```python
from build123d import *

# Parameters (mm, degrees)
BOSS_EXTRU_1_DEPTH = 8


with BuildPart() as part:
    # Esquisse2 → Boss.-Extru.1 (new body)
    with BuildSketch(Plane.XY):
        with BuildLine():
            Line((-234, 77.582220472), (250, 77.582220472))
            Line((250, 77.582220472), (250, 68.582220472))
            Line((250, 68.582220472), (230.972064578, 68.582220472))
            ThreePointArc((230.972064578, 68.582220472), (228.850744234, 68.582220472), (228.850744234, 66.460900128))
            Line((228.850744234, 66.460900128), (228.850744234, 60.582220472))
            Line((228.850744234, 60.582220472), (218.850744234, 60.582220472))
            Line((218.850744234, 60.582220472), (218.850744234, 66.460900128))
            ThreePointArc((218.850744234, 66.460900128), (218.850744234, 68.582220472), (216.729423891, 68.582220472))
            Line((216.729423891, 68.582220472), (115.787517246, 68.582220472))
            ThreePointArc((115.787517246, 68.582220472), (113.666196902, 68.582220472), (113.666196902, 66.460900128))
            Line((113.666196902, 66.460900128), (113.666196902, 60.582220472))
            Line((113.666196902, 60.582220472), (63.666196902, 60.582220472))
            Line((63.666196902, 60.582220472), (63.666196902, 66.460900128))
            ThreePointArc((63.666196902, 66.460900128), (63.666196902, 68.582220472), (61.544876559, 68.582220472))
            Line((61.544876559, 68.582220472), (-45.544876559, 68.582220472))
            ThreePointArc((-45.544876559, 68.582220472), (-47.666196902, 68.582220472), (-47.666196902, 66.460900128))
            Line((-47.666196902, 66.460900128), (-47.666196902, 60.582220472))
            Line((-47.666196902, 60.582220472), (-97.666196902, 60.582220472))
            Line((-97.666196902, 60.582220472), (-97.666196902, 66.460900128))
            ThreePointArc((-97.666196902, 66.460900128), (-97.666196902, 68.582220472), (-99.787517246, 68.582220472))
            Line((-99.787517246, 68.582220472), (-200.729423891, 68.582220472))
            ThreePointArc((-200.729423891, 68.582220472), (-202.850744234, 68.582220472), (-202.850744234, 66.460900128))
            Line((-202.850744234, 66.460900128), (-202.850744234, 60.582220472))
            Line((-202.850744234, 60.582220472), (-212.850744234, 60.582220472))
            Line((-212.850744234, 60.582220472), (-212.850744234, 66.460900128))
            ThreePointArc((-212.850744234, 66.460900128), (-212.850744234, 68.582220472), (-214.972064578, 68.582220472))
            Line((-214.972064578, 68.582220472), (-234, 68.582220472))
            Line((-234, 68.582220472), (-234, 77.582220472))
        make_face()
    extrude(amount=BOSS_EXTRU_1_DEPTH)


solid = part.part
```
Build history of the part. All positions in model axes, mm. A direction names the side the tool comes from. Round coordinates to 2 decimals unless told otherwise and drop trailing zeros. Loops run counter-clockwise (first coordinate to the right, second up) from the corner with the lowest first, then second, coordinate; pieces in that order, holes last.
Item 1: Drill centre lines: line 1 along X through (y, z) = (63, 2.25); line 2 along Y through (x, z) = (204.5, 3). Where is each one in solid material? Low to high.
Item 2: Pin check, flat tips, straight feed: P1, Ø3, axis at x = 165, z = 7, coming from the -Y side; P2, Ø3, axis at x = 41.5, y = 67, coming from the +Z side; P3, Ø4.5, axis at y = 63.5, z = 5.5, coming from the +X side; P4, Ø1.8, axis at y = 63, z = 3.5, coming from the -X side. Stop position of each tip, or through.
Item 3: Which spindle directions (+Z, -Z, +X, -X, +Y, -Y) get a long thin tool onto all of the face, cutting with end or side? Do faces 4 (the face through (-224, 68.582, 4)), 5 (the face through (5, 77.582, 4)), 6 (the face through (-150, 68.582, 4)). Say none if no direction does.
Item 4: Saw through at A-A (z = 4.5). List the corners of the cut face in (x, y).
Item 5: Two-plate mould, pull along X, no slides. Class faces 1 (the face through (-234, 73, 4)), 2 (the face through (241, 68.582, 4)), 3 (the face through (9, 68.582, 4)): released by +X, released by -X, zero draft, split by the parting line, or undercut.
Item 6: Saw through at B-B (x = 150.5). List the corners of the cut face in (y, z), then the cut area to 3 significant figures.
Worked answers:
1. line 1: x = -212.85 to -202.85, -97.67 to -47.67, 63.67 to 113.67, 218.85 to 228.85
1. line 2: y = 68.58 to 77.58
2. P1: stops at y = 68.58
2. P2: passes through
2. P3: stops at x = 228.85
2. P4: stops at x = -212.85
3. face 4: +Z, -Z, -X, -Y
3. face 5: +Z, -Z, +X, -X, +Y
3. face 6: +Z, -Z, -Y
4. outline: (-234, 68.58) - (-214.97, 68.58) arc R1.5 cw to (-212.85, 66.46) - (-212.85, 60.58) - (-202.85, 60.58) - (-202.85, 66.46) arc R1.5 cw to (-200.73, 68.58) - (-99.79, 68.58) arc R1.5 cw to (-97.67, 66.46) - (-97.67, 60.58) - (-47.67, 60.58) - (-47.67, 66.46) arc R1.5 cw to (-45.54, 68.58) - (61.54, 68.58) arc R1.5 cw to (63.67, 66.46) - (63.67, 60.58) - (113.67, 60.58) - (113.67, 66.46) arc R1.5 cw to (115.79, 68.58) - (216.73, 68.58) arc R1.5 cw to (218.85, 66.46) - (218.85, 60.58) - (228.85, 60.58) - (228.85, 66.46) arc R1.5 cw to (230.97, 68.58) - (250, 68.58) - (250, 77.58) - (-234, 77.58) - close
5. face 1: released by -X
5. face 2: zero draft
5. face 3: undercut
6. outline: (68.58, 0) - (77.58, 0) - (77.58, 8) - (68.58, 8) - close
6. area: 72.0 mm2
